Can you work these out from the model? Positions are in its coordinate system, mm. Face numbers are marked on the shaded views. A direction names the side the tool comes from. Give positions to 0.01 mm unless a question says otherwise; leave off trailing zeros. Loops run counter-clockwise (first coordinate to the right, second up) from the corner with the lowest first, then second, coordinate; pieces in that order, holes last. Notation, with made-up numbers: (62, 35.25) -> (93, 35.25) arc R23 ccw to (93, 66.25) -> close; hole circle Ø11 at (-7, 77.5). An arc over 180 degrees is marked (long way). Use CSV: the item, a comma, the result in double quotes.
from build123d import *

# Parameters (mm, degrees)
F0_W     = 57.15
F0_H     = 44.45
F1_DEPTH = 25.4
F3_DEPTH = 12.7
F4_R     = 12.7
F5_DEPTH = 12.701
F7_DEPTH = 25.4


with BuildPart() as f1:
    # F0 (on Front) → F1 (new body)
    with BuildSketch(Plane.XZ):
        with Locations((-28.575, 22.225)):
            Rectangle(F0_W, F0_H)
    extrude(amount=F1_DEPTH)

    # F2 (on face) → F3 (cut)
    with BuildSketch(Plane.XZ.offset(25.4)):
        Polygon((0, 44.45), (-38.1, 44.45), (-12.7, 0), (0, 0), align=None)
    extrude(amount=-F3_DEPTH, mode=Mode.SUBTRACT)

    # F4 (on face) → F5 (cut, through all)
    with BuildSketch(Plane.XZ.offset(12.7)):
        with Locations((-31.75, 25.4)):
            Circle(F4_R)
    extrude(amount=F5_DEPTH, mode=Mode.SUBTRACT)

    # F6 (on face) → F7 (cut)
    with BuildSketch(Plane.XZ.offset(12.7)):
        with BuildLine():
            Line((-34.321148, 37.837009), (-34.341116, 37.871952))
            ThreePointArc((-34.341116, 37.871952), (-42.809914, 19.080049), (-22.320423, 16.83574))
            Line((-22.320423, 16.83574), (-22.34039, 16.870683))
            ThreePointArc((-22.34039, 16.870683), (-42.776688, 19.099035), (-34.321148, 37.837009))
        make_face()
        with BuildLine():
            ThreePointArc((-22.320423, 16.83574), (-19.867661, 20.809412), (-19.011732, 25.4))
            ThreePointArc((-19.011732, 25.4), (-23.71081, 35.281037), (-34.341116, 37.871952))
            Line((-34.341116, 37.871952), (-34.321148, 37.837009))
            ThreePointArc((-34.321148, 37.837009), (-42.776688, 19.099035), (-22.34039, 16.870683))
            Line((-22.34039, 16.870683), (-22.320423, 16.83574))
        make_face()
    extrude(amount=-F7_DEPTH, mode=Mode.SUBTRACT)


solid = f1.part
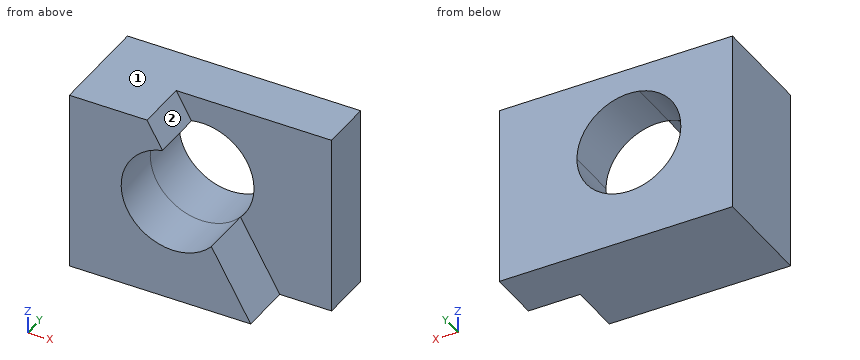
(1) If we section it at A-A, the plane y = -8: Write out the boundary of the cut face in (x, z), then the cut area to 3 significant figures.
Answer sheet:
outline,"(-57.15, 0) -> (0, 0) -> (0, 44.45) -> (-57.15, 44.45) -> close; hole (-22.32, 16.84) arc R12.74 ccw to (-19.01, 25.4) arc R12.74 ccw (long way) to start"
area,"2,030 mm2"
(2) Which directions (+Z, -Z, +X, -X, +Y, -Y) give clear straight access to the entire face, cutting with the end or side of a thin tool? Please do the marked faces 1 and 2.
Answer sheet:
face 1,"+Z, +X, -X, +Y, -Y"
face 2,"+Z, +X, -Y"
(3) If we section it at D-D, the plane x = -11: Write out the boundary of the cut face in (y, z), then the cut area to 3 significant figures.
Answer sheet:
outline,"(-12.7, 0) -> (0, 0) -> (0, 44.45) -> (-12.7, 44.45) -> close"
area,"565 mm2"
(4) If I drill on L1, parallel to Z at x = -31.75, y = -5; L2, parallel to X at y = -3.25, z = 25.4; L3, parallel to Y at x = -3.5, z = 27, over which ranges is the centre line in solid material (lowest first)? Write a range as from..to.
Answer sheet:
L1,"z = 0..12.66, 38.14..44.45"
L2,"x = -57.15..-44.49, -19.01..0"
L3,"y = -12.7..0"
(5) Will this pin go through, and if not, where does the flat tip stop? pin 1 Ø5 at (y, z) = (-20, 5) entering from +X.
Answer sheet:
pin 1,"stops at x = -14.13"
